Job drawing, mm, ordinate dimensions from the low corner. One solid piece. A direction names the side the tool comes from. Give positions to 0.01 mm unless a question says otherwise; leave off trailing zeros. Order: outer loops, then holes, each group sorted by start corner. A loop starts at its lowest first (then second) coordinate and runs counter-clockwise, first axis right, second up. Notation, with made-up numbers: M 10,-34.75 L 39,-34.75 A15 cw 39,-23.75 Z; hole C 33,31 d4. An arc over 180 degrees is marked long. Use CSV: the item, a comma, the result in double quotes. Start each with the question number.
Item 1: Band-saw the part on B-B on z = 30.1. Write the cut outline in (x, y).
Item 2: Band-saw the part on C-C on y = 1.5. Write the cut outline in (x, z).
Item 3: Two-plate mould, pull along Z, no slides. Class the marked faces 4, 5 and 6: pulls with the +Z half, pulls with the -Z half, needs draft (parallel to the pull), parting line crosses it, or undercut.
Item 4: Which spindle directions (+Z, -Z, +X, -X, +Y, -Y) get a long thin tool onto all of the face, cutting with end or side? Do the marked faces 1, 2 and 3. Say none if no direction does.
Item 5: Band-saw the part on A-A on x = 30.1. Write the cut outline in (y, z), plus the area to 3 significant figures.
Item 6: Band-saw the part on D-D on z = 43. Write the cut outline in (x, y), plus the area to 3 significant figures.
Item 7: Wall check: line 1 along Z through (x, y) = (30.1, 3.85); line 2 along X through (y, z) = (4, 28); line 3 along X through (y, z) = (11.75, 29). Give the ranges that are in metal, low to high.
Item 8: Pin check, flat tips, straight feed: P1, Ø3, axis at x = 49, z = 28.5, coming from the +Y side; P2, Ø1, axis at y = 14.5, z = 20.5, coming from the +X side; P3, Ø1, axis at y = 5.5, z = 42, coming from the -X side. Stop position of each tip, or through.
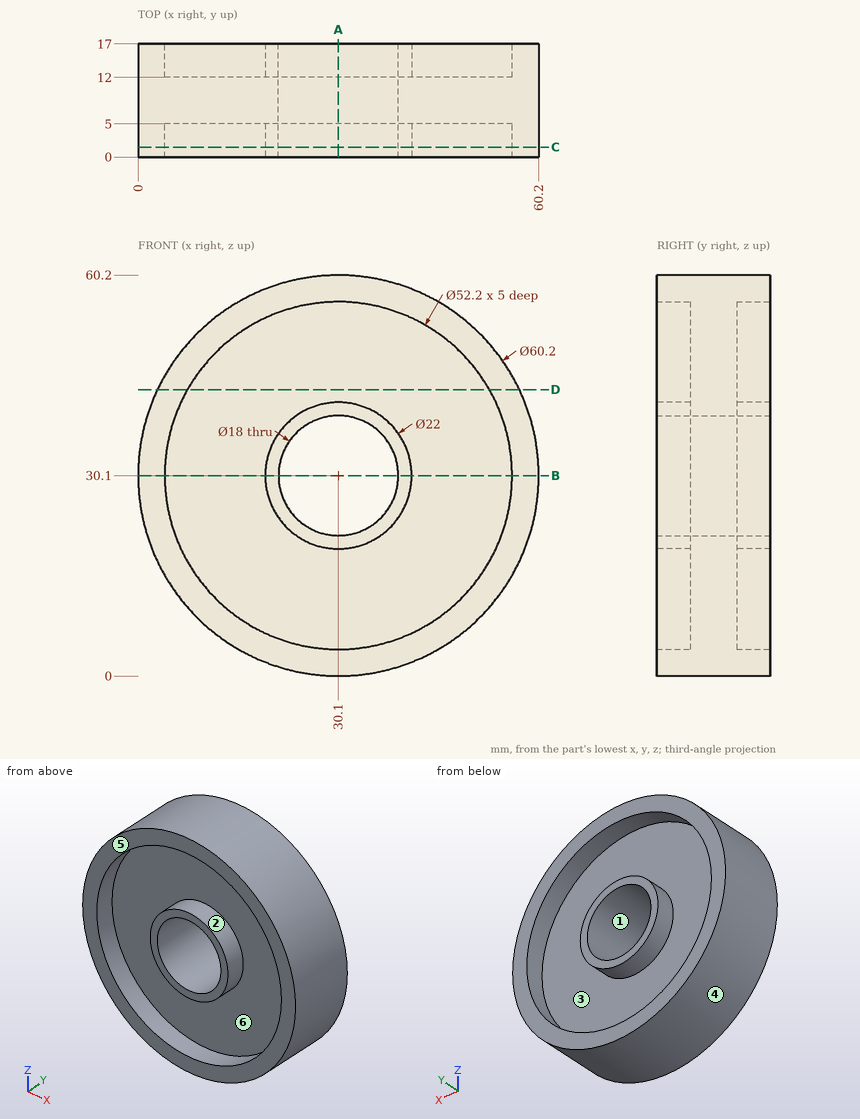
Model answer:
1,outline,"M 0,0 L 4,0 L 4,5 L 19.1,5 L 19.1,0 L 21.1,0 L 21.1,17 L 19.1,17 L 19.1,12 L 4,12 L 4,17 L 0,17 Z; M 39.1,0 L 41.1,0 L 41.1,5 L 56.2,5 L 56.2,0 L 60.2,0 L 60.2,17 L 56.2,17 L 56.2,12 L 41.1,12 L 41.1,17 L 39.1,17 Z"
2,outline,"C 30.1,30.1 d60.2; C 30.1,30.1 d22; hole C 30.1,30.1 d52.2; hole C 30.1,30.1 d18"
3,face 4,"parting line crosses it"
3,face 5,"needs draft"
3,face 6,"undercut"
4,face 1,"+Y, -Y"
4,face 2,"-Y"
4,face 3,"+Y"
5,outline,"M 0,0 L 17,0 L 17,4 L 12,4 L 12,19.1 L 17,19.1 L 17,21.1 L 0,21.1 L 0,19.1 L 5,19.1 L 5,4 L 0,4 Z; M 0,39.1 L 17,39.1 L 17,41.1 L 12,41.1 L 12,56.2 L 17,56.2 L 17,60.2 L 0,60.2 L 0,56.2 L 5,56.2 L 5,41.1 L 0,41.1 Z"
5,area,"415 mm^2"
6,outline,"M 2.9,0 L 7.41,0 L 7.41,5 L 52.79,5 L 52.79,0 L 57.3,0 L 57.3,17 L 52.79,17 L 52.79,12 L 7.41,12 L 7.41,17 L 2.9,17 Z"
6,area,"471 mm^2"
7,line 1,"z = 0 to 4, 19.1 to 21.1, 39.1 to 41.1, 56.2 to 60.2"
7,line 2,"x = 0.07 to 4.08, 19.3 to 21.35, 38.85 to 40.9, 56.12 to 60.13"
7,line 3,"x = 0.02 to 21.17, 39.03 to 60.18"
8,P1,"stops at y = 12"
8,P2,"stops at x = 58.79"
8,P3,"stops at x = 2.24"
